```python
from build123d import *

# Parameters (mm, degrees)
BOX_W        = 100
BOX_H        = 16
BOX_DEPTH    = 1
BOX001_W     = 100
BOX001_H     = 12
BOX001_DEPTH = 1


with BuildPart() as f_16mm:
    # Box → Box (new body)
    with BuildSketch(Plane.XY.offset(1)):
        with Locations((50, 8)):
            Rectangle(BOX_W, BOX_H)
    extrude(amount=BOX_DEPTH)


with BuildPart() as k8200_profile:
    # Box001 → Box001 (new body)
    with BuildSketch(Plane(origin=(0, 2, 0), x_dir=(1, 0, 0), z_dir=(0, 0, 1))):
        with Locations((50, 6)):
            Rectangle(BOX001_W, BOX001_H)
    extrude(amount=BOX001_DEPTH)

    # Fusion: union 16mm
    add(f_16mm.part)


solid = k8200_profile.part
```
For this review, take the finished solid that the model builds, in its own axes (mm). A direction names the side the tool comes from. Coordinates: 2 decimals unless noted, no trailing zeros. Loops run counter-clockwise (first coordinate to the right, second up) from the corner with the lowest first, then second, coordinate; pieces in that order, holes last.
1. Add section B-B, the plane z = 0.55. Give the boundary of the cut face in (x, y), then the cut area to 3 significant figures.
2. For faces 1 (the flat face through (0, 8, 1)), 2 (the flat face through (49, 15, 1)), 3 (the flat face through (49, 1, 1)), list the 3-axis set-ups (+Z, -Z, +X, -X, +Y, -Y) from which the entire face can be reached by the end or side of a thin tool; tool diameter is ignored.
3. Add section A-A, the plane x = 88. Give the boundary of the cut face in (y, z).
4. Insertion check: P1, Ø0.5, axis at x = 51, z = 0.5, coming from the -Y side; P2, Ø0.6, axis at x = 70, y = 15, coming from the -Z side. Each pin has a flat end and moves straight along its axis. Give the tip position at first contact, or say it passes through.
5. For line 1 (Z direction, x = 7.5, y = 1.5); line 2 (Y direction, x = 74, z = 0.65), list the stretches that pass through material, from the lowest coordinate up.
Result:
1. outline: (0, 2) - (100, 2) - (100, 14) - (0, 14) - close
1. area: 1,200 mm2
2. face 1: +Z, -Z, -X, +Y, -Y
2. face 2: -Z, +X, -X, +Y
2. face 3: -Z, +X, -X, -Y
3. outline: (0, 1) - (2, 1) - (2, 0) - (14, 0) - (14, 1) - (16, 1) - (16, 2) - (0, 2) - close
4. P1: stops at y = 2
4. P2: stops at z = 1
5. line 1: z = 1 to 2
5. line 2: y = 2 to 14
